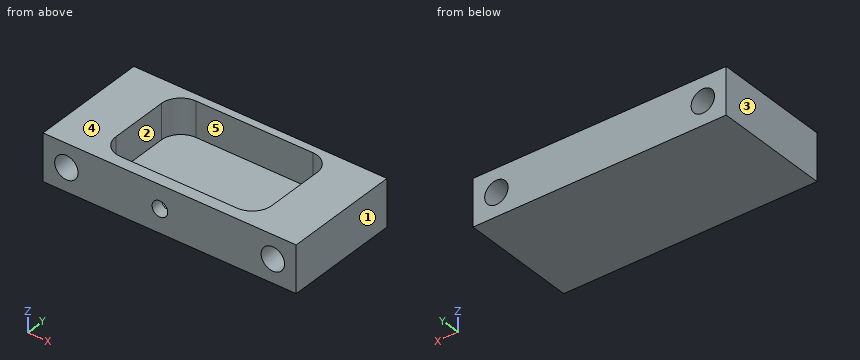
from build123d import *

# Parameters (mm, degrees)
F0_W     = 65
F0_H     = 30
F1_DEPTH = 12
F4_D     = 6
F5_D     = 6
F6_W     = 40
F6_H     = 25
F7_DEPTH = 9
F8_R     = 5
F9_D     = 4
F9_DEPTH = 7
F9_TIP   = 1.2017212381


# Not quite as in the source:
# - a feature names something its author has since deleted; it is built from what else it names


with BuildPart() as f1:
    # F0 (on Top) → F1 (new body)
    with BuildSketch(Plane.XY):
        with Locations((10.1498100485, -9.411229075)):
            Rectangle(F0_W, F0_H)
    extrude(amount=F1_DEPTH)

    # F4 (through all)
    with Locations(Plane.XZ.offset(24.411229075)):
        with Locations((36.6498100485, 6)):
            Hole(F4_D / 2)

    # F5 (through all)
    with Locations(Plane.XZ.offset(24.411229075)):
        with Locations((-16.3501899515, 6)):
            Hole(F5_D / 2)

    # F6 (on face) → F7 (cut)
    with BuildSketch(Plane.XY.offset(12)):
        with Locations((10.1498100485, -8.911229075)):
            Rectangle(F6_W, F6_H)
    extrude(amount=-F7_DEPTH, mode=Mode.SUBTRACT)

    # F8
    f8_edges = [f1.edges().sort_by_distance(p)[0] for p in [
        (-9.85019, 3.588771, 7.5),
        (-9.85019, -21.411229, 7.5),
        (30.14981, 3.588771, 7.5),
        (30.14981, -21.411229, 7.5),
    ]]
    fillet(f8_edges, radius=F8_R)

    # F9
    with Locations(Plane.XZ.offset(24.411229075)):
        with Locations((7.6498100485, 6)):
            Hole(F9_D / 2, depth=F9_DEPTH)
            with Locations((0, 0, -(F9_DEPTH + F9_TIP / 2))):  # 118° drill point
                Cone(0, F9_D / 2, F9_TIP, mode=Mode.SUBTRACT)


solid = f1.part
Check sheet for the modelled part. Datum: model origin and axes. Units: mm. Face numbers are marked on the shaded views. A direction names the side the tool comes from. Round coordinates to 2 decimals unless told otherwise and drop trailing zeros. Loops run counter-clockwise (first coordinate to the right, second up) from the corner with the lowest first, then second, coordinate; pieces in that order, holes last. Notation, with made-up numbers: (36.5, 31.5) -> (78.5, 31.5) arc R9 ccw to (78.5, 48.5) -> close; hole circle Ø4 at (-17.5, -39.5). An arc over 180 degrees is marked (long way). Put each result on its own line as item: value. Start each with the question number.
1. Scan lines: probe 1 along Y at (x, z) = (25, 8); probe 2 along X at (y, z) = (-4, 10); probe 3 along X at (y, z) = (-21.5, 4.75). Record each from-to range of solid material in increasing order.
2. Section check A-A (z = 10). Enter the section's corners in (x, y), plus the area to 3 significant figures.
3. Section check B-B (y = -6). Enter the section's corners in (x, z), plus the area to 3 significant figures.
4. Section check D-D (z = 6). Enter the section's corners in (x, y).
5. Draft check along X on the marked faces 3, 4 and 5. Enter one of: +X half, -X half, draft (parallel to the pull), parting line (faces both ways), or undercut.
6. Gauge pin test, flat end, axial feed: pin 1 (1 mm diameter, centred on x = 8, y = -7.5, fed in from +Z). Record the tip position at first contact, or that the pin passes through.
7. Section check C-C (x = 36). Enter the section's corners in (y, z).
8. Access from +Z, -Z, +X, -X, +Y, -Y to the whole of each face (thin tool, end or side, straight path). Record for the marked faces 1 and 2.
Findings:
1. probe 1: y = -24.41 to -21.41, 3.59 to 5.59
1. probe 2: x = -22.35 to -9.85, 30.15 to 42.65
1. probe 3: x = -22.35 to -19.08, -13.62 to 6.09, 9.21 to 33.92, 39.38 to 42.65
2. outline: (-22.35, -24.41) -> (42.65, -24.41) -> (42.65, 5.59) -> (-22.35, 5.59) -> close; hole (-9.85, -16.41) arc R5 ccw to (-4.85, -21.41) -> (25.15, -21.41) arc R5 ccw to (30.15, -16.41) -> (30.15, -1.41) arc R5 ccw to (25.15, 3.59) -> (-4.85, 3.59) arc R5 ccw to (-9.85, -1.41) -> close
2. area: 971 mm^2
3. outline: (-22.35, 0) -> (42.65, 0) -> (42.65, 12) -> (30.15, 12) -> (30.15, 3) -> (-9.85, 3) -> (-9.85, 12) -> (-22.35, 12) -> close; hole circle Ø6 at (-16.35, 6); hole circle Ø6 at (36.65, 6)
3. area: 363 mm^2
4. outline: (-22.35, -24.41) -> (-19.35, -24.41) -> (-19.35, 5.59) -> (-22.35, 5.59) -> close; (-13.35, -24.41) -> (5.65, -24.41) -> (5.65, -21.41) -> (-4.85, -21.41) arc R5 cw to (-9.85, -16.41) -> (-9.85, -1.41) arc R5 cw to (-4.85, 3.59) -> (25.15, 3.59) arc R5 cw to (30.15, -1.41) -> (30.15, -16.41) arc R5 cw to (25.15, -21.41) -> (9.65, -21.41) -> (9.65, -24.41) -> (33.65, -24.41) -> (33.65, 5.59) -> (-13.35, 5.59) -> close; (39.65, -24.41) -> (42.65, -24.41) -> (42.65, 5.59) -> (39.65, 5.59) -> close
5. face 3: -X half
5. face 4: draft
5. face 5: undercut
6. pin 1: stops at z = 3
7. outline: (-24.41, 0) -> (5.59, 0) -> (5.59, 3.07) -> (-24.41, 3.07) -> close; (-24.41, 8.93) -> (5.59, 8.93) -> (5.59, 12) -> (-24.41, 12) -> close
8. face 1: +Z, -Z, +X, +Y, -Y
8. face 2: +Z
